Source: three-view drawing plus pictorial views. Frame: mm from the lowest corner of the part. A direction names the side the tool comes from. Give positions to 0.01 mm unless a question says otherwise; leave off trailing zeros. Order: outer loops, then holes, each group sorted by start corner. A loop starts at its lowest first (then second) coordinate and runs counter-clockwise, first axis right, second up. Notation, with made-up numbers: M -34,-26 L 8,-26 A14 cw 8,-21 Z; hole C 75.5,85.5 d3. An arc over 180 degrees is marked long. Use CSV: the item, a comma, the result in double quotes. Start each with the question number.
1. Section query D-D, the plane z = 1. Return the cut outline in (x, y), plus the area to 3 significant figures.
2. Reachability of the marked faces 1, 2 and 3 from +Z, -Z, +X, -X, +Y, -Y: full face, straight path, thin tool, end or side. Return the list, or none.
3. Section query C-C, the plane y = 6. Return the cut outline in (x, z), plus the area to 3 significant figures.
4. Line query: line 1 along X through (y, z) = (13.85, 5.8); line 2 along Y through (x, z) = (23.25, 7.25); line 3 along X through (y, z) = (4, 1). Output: solid intervals per line, ascending. Write a range as [from, to].
5. Section query B-B, the plane x = 15.75. Return the cut outline in (y, z), plus the area to 3 significant figures.
6. Section query A-A, the plane x = 27.75. Return the cut outline in (y, z), plus the area to 3 significant figures.
7. Pin query (flat end, axial travel): P1, Ø6, axis at y = 6.5, z = 4, coming from the -X side; P2, Ø2, axis at x = 27.5, z = 7.5, coming from the +Y side; P3, Ø1.1, axis at y = 15.5, z = 6, coming from the +X side; P4, Ø4, axis at y = 16, z = 3.5, coming from the -X side. Return the tip coordinate at first contact, or that it passes through.
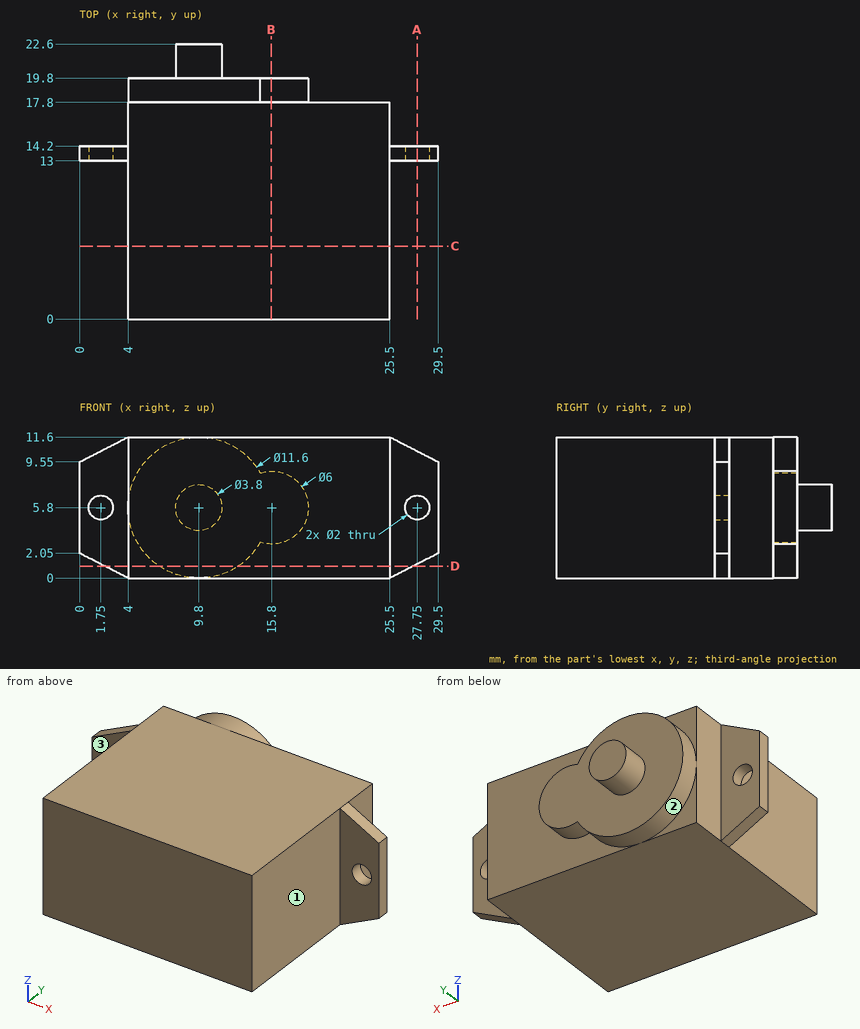
Result set:
1,outline,"M 2.05,13 L 4,13 L 4,0 L 25.5,0 L 25.5,13 L 27.45,13 L 27.45,14.2 L 25.5,14.2 L 25.5,17.8 L 13.06,17.8 L 13.06,19.8 L 6.54,19.8 L 6.54,17.8 L 4,17.8 L 4,14.2 L 2.05,14.2 Z"
1,area,"400 mm2"
2,face 1,"+Z, -Z, +X, -Y"
2,face 2,"+Y"
2,face 3,"+Z, -Z, -X, -Y"
3,outline,"M 4,0 L 25.5,0 L 25.5,11.6 L 4,11.6 Z"
3,area,"249 mm2"
4,line 1,"[0, 0.75], [2.75, 26.75], [28.75, 29.5]"
4,line 2,"[0, 17.8]"
4,line 3,"[4, 25.5]"
5,outline,"M 0,0 L 17.8,0 L 17.8,2.8 L 19.8,2.8 L 19.8,8.8 L 17.8,8.8 L 17.8,11.6 L 0,11.6 Z"
5,area,"218 mm2"
6,outline,"M 13,1.15 L 14.2,1.15 L 14.2,4.8 L 13,4.8 Z; M 13,6.8 L 14.2,6.8 L 14.2,10.45 L 13,10.45 Z"
6,area,"8.75 mm2"
7,P1,"x = 4"
7,P2,"y = 14.2"
7,P3,"x = 25.5"
7,P4,"x = 0"
